```python
from build123d import *

# Parameters (mm, degrees)
SKETCH_1_W              = 55
SKETCH_1_H              = 20
EXTRUDE_1_DEPTH         = 16
SKETCH_2_R              = 4
CUT_EXTRUDE_1_DEPTH     = 18
HOLE_WIZARD_6_5_6_5_1_D = 6.5


with BuildPart() as part:
    # Эскиз1 → Бобышка-Вытянуть1 (new body)
    with BuildSketch(Plane.XY):
        Rectangle(SKETCH_1_W, SKETCH_1_H)
    extrude(amount=EXTRUDE_1_DEPTH)

    # Эскиз2 → Вырез-Вытянуть1 (cut)
    with BuildSketch(Plane.XY.offset(16)):
        with Locations((-6, 0)):
            Circle(SKETCH_2_R)
    extrude(amount=-CUT_EXTRUDE_1_DEPTH, mode=Mode.SUBTRACT)

    # Диаметр отверстия Ø6.5 (6.5)1 (through all)
    with Locations(Plane(origin=(0, 10, 0), x_dir=(1, 0, 0), z_dir=(0, 1, 0))):
        with Locations((19.8, -8), (-19.8, -8)):
            Hole(HOLE_WIZARD_6_5_6_5_1_D / 2)


solid = part.part
```
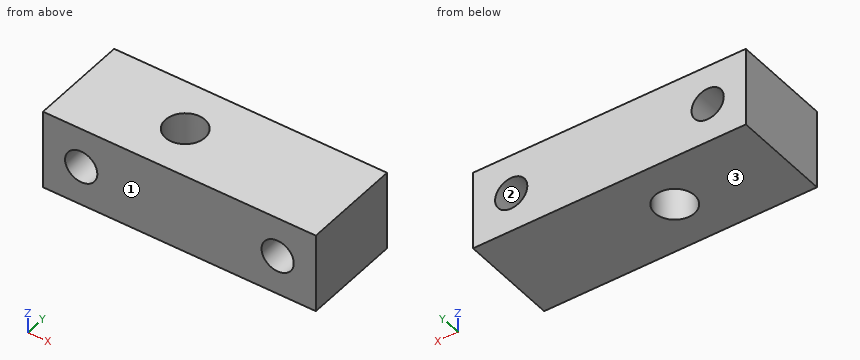
Here's how the part is built. I have some questions about the finished solid (model axes, mm). Face numbers are marked on the shaded views. Give positions to 0.01 mm unless a question says otherwise; leave off trailing zeros. Order: outer loops, then holes, each group sorted by start corner. A loop starts at its lowest first (then second) coordinate and runs counter-clockwise, first axis right, second up. Notation, with made-up numbers: (76, 33) -> (134, 33) arc R16 ccw to (134, 41) -> close; hole circle Ø9 at (-29, 55.5). An arc over 180 degrees is marked (long way). Use CSV: the item, a comma, the result in double quotes. Start each with the question number.
Item 1: Suppose I cut it at C-C (x = -7.5). List the corners of the cut face in (y, z) for me, and give its area (3 significant figures).
Item 2: Suppose I cut it at D-D (y = -6.25). List the corners of the cut face in (x, z) for me.
Item 3: If I drill on probe 1 along X at (y, z) = (4.75, 8); probe 2 along Z at (x, y) = (-19.8, -1); probe 3 along Y at (x, z) = (-6, 10.5), over which ranges is the centre line in solid material (lowest first)? Write a range as [from, to].
Item 4: Suppose I cut it at B-B (z = 8). List the corners of the cut face in (x, y) for me.
Item 5: Suppose I cut it at A-A (y = 0). List the corners of the cut face in (x, z) for me.
Item 6: Thinking about a two-plate mould opening in Z: for the marked faces 1, 2 and 3, which applies, pulls with the +Z half, pulls with the -Z half, needs draft (parallel to the pull), parting line crosses it, or undercut?
Answer block:
1,outline,"(-10, 0) -> (-3.71, 0) -> (-3.71, 16) -> (-10, 16) -> close; (3.71, 0) -> (10, 0) -> (10, 16) -> (3.71, 16) -> close"
1,area,"201 mm^2"
2,outline,"(-27.5, 0) -> (27.5, 0) -> (27.5, 16) -> (-27.5, 16) -> close; hole circle Ø6.5 at (-19.8, 8); hole circle Ø6.5 at (19.8, 8)"
3,probe 1,"x = [-27.5, -23.05], [-16.55, 16.55], [23.05, 27.5]"
3,probe 2,"z = [0, 4.75], [11.25, 16]"
3,probe 3,"y = [-10, -4], [4, 10]"
4,outline,"(-27.5, -10) -> (-23.05, -10) -> (-23.05, 10) -> (-27.5, 10) -> close; (-16.55, -10) -> (16.55, -10) -> (16.55, 10) -> (-16.55, 10) -> close; (23.05, -10) -> (27.5, -10) -> (27.5, 10) -> (23.05, 10) -> close; hole circle Ø8 at (-6, 0)"
5,outline,"(-27.5, 0) -> (-10, 0) -> (-10, 16) -> (-27.5, 16) -> close; (-2, 0) -> (27.5, 0) -> (27.5, 16) -> (-2, 16) -> close; hole circle Ø6.5 at (-19.8, 8); hole circle Ø6.5 at (19.8, 8)"
6,face 1,"needs draft"
6,face 2,"undercut"
6,face 3,"pulls with the -Z half"
